from build123d import *

# Parameters (mm, degrees)
F1_DEPTH = 8
F2_R     = 1.5
F3_DEPTH = 3.8920101006
F4_R     = 0.5


with BuildPart() as f1:
    # F0 (on Front) → F1 (new body)
    with BuildSketch(Plane.XZ):
        with BuildLine():
            Line((3, 14.471053486), (0, 14.471053486))
            Line((0, 14.471053486), (0, -5.528946514))
            Line((0, -5.528946514), (3, -5.528946514))
            Line((3, -5.528946514), (3, -3.3778412531))
            ThreePointArc((3, -3.3778412531), (3.7830427709, -0.6913432113), (5.8869086913, 1.1536976821))
            Line((5.8869086913, 1.1536976821), (10.3150881731, 3.2185916862))
            Line((10.3150881731, 3.2185916862), (10.3150881731, -0.0229635164))
            Line((10.3150881731, -0.0229635164), (16.2366852164, -0.0229635164))
            Line((16.2366852164, -0.0229635164), (16.2366852164, 11.9770364836))
            Line((16.2366852164, 11.9770364836), (10.3150881731, 11.9770364836))
            Line((10.3150881731, 11.9770364836), (10.3150881731, 8.735481281))
            Line((10.3150881731, 8.735481281), (4.7242360053, 6.1284240995))
            ThreePointArc((4.7242360053, 6.1284240995), (3.5608002487, 6.2046797078), (3, 7.2268835811))
            Line((3, 7.2268835811), (3, 14.471053486))
        make_face()
    extrude(amount=F1_DEPTH)

    # F2 (on Right) → F3 (cut, through all)
    with BuildSketch(Plane.YZ):
        with Locations((-4, -2.028946514)):
            Circle(F2_R)
        with Locations((-4, 10.971053486)):
            Circle(F2_R)
    extrude(amount=F3_DEPTH, mode=Mode.SUBTRACT)

    # F4
    f4_edges = [f1.edges().sort_by_distance(p)[0] for p in [
        (7.519662, 0, 7.431953),
        (8.100998, 0, 2.186145),
        (7.519662, -8, 7.431953),
        (8.100998, -8, 2.186145),
    ]]
    fillet(f4_edges, radius=F4_R)


solid = f1.part
Model file for the job. Use its own axes, mm. A direction names the side the tool comes from. Give positions to 0.01 mm unless a question says otherwise; leave off trailing zeros. Write each loop counter-clockwise with the first axis right and the second up, starting at its lowest first coordinate (ties: lowest second). Pieces come first, ordered by that corner, then holes. Notation, with made-up numbers: (28, 41.25) - (55, 41.25) arc R22 ccw to (55, 73.25) - close; hole circle Ø3 at (58, -21.5). An arc over 180 degrees is marked (long way). Answer as CSV lines item,"result".
1. Band-saw the part on D-D (x = 2.75). Count the separate pieces of the cut face and the enclosed holes in it, and give its area (3 significant figures).
Responses:
separate pieces,"1"
enclosed holes,"2"
area,"144 mm2"
2. Band-saw the part on B-B (z = -3.75). Write the cut outline in (x, y).
Responses:
outline,"(0, -8) - (2.5, -8) arc R0.5 ccw to (3, -7.5) - (3, -0.5) arc R0.5 ccw to (2.5, 0) - (0, 0) - close"
3. Band-saw the part on A-A (y = -4). Write the cut outline in (x, z), and give its area (3 significant figures).
Responses:
outline,"(0, -5.53) - (3, -5.53) - (3, -3.53) - (0, -3.53) - close; (0, -0.53) - (3.89, -0.53) arc R5 cw to (5.89, 1.15) - (10.32, 3.22) - (10.32, -0.02) - (16.24, -0.02) - (16.24, 11.98) - (10.32, 11.98) - (10.32, 8.74) - (4.72, 6.13) arc R1.21 cw to (3, 7.23) - (3, 9.47) - (0, 9.47) - close; (0, 12.47) - (3, 12.47) - (3, 14.47) - (0, 14.47) - close"
area,"155 mm2"
4. Drill centre lines: L1, parallel to Z at x = 2.1, y = -4; L2, parallel to X at y = -6.5, z = 10.5; L3, parallel to Z at x = 15.75, y = -2.25. Where is each one in solid material? Low to high. Write a range as [from, to].
Responses:
L1,"z = [-5.53, -3.53], [-0.53, 9.47], [12.47, 14.47]"
L2,"x = [0, 3], [10.32, 16.24]"
L3,"z = [-0.02, 11.98]"
5. Band-saw the part on C-C (y = -5.75). Write the cut outline in (x, z), and give its area (3 significant figures).
Responses:
outline,"(0, -5.53) - (3, -5.53) - (3, -3.38) arc R5 cw to (5.89, 1.15) - (10.32, 3.22) - (10.32, -0.02) - (16.24, -0.02) - (16.24, 11.98) - (10.32, 11.98) - (10.32, 8.74) - (4.72, 6.13) arc R1.21 cw to (3, 7.23) - (3, 14.47) - (0, 14.47) - close"
area,"174 mm2"
6. 3-axis set-ups, long thin cutter, end or side, ignore diameter. For faces 4 (the face through (13, -4, 11.977)), 5 (the face through (13, -4, -0.023)), 6 (the face through (3, -6, 11)): which of +Z, -Z, +X, -X, +Y, -Y reach the whole face in a straight line?
Responses:
face 4,"+Z, +X, +Y, -Y"
face 5,"-Z, +X, +Y, -Y"
face 6,"+Z, +Y, -Y"
7. Pin check, flat tips, straight feed: pin 1 (3.5 mm diameter, centred on y = -4, z = 10.97, fed in from -X); pin 2 (4 mm diameter, centred on x = 13, y = -6, fed in from -Z); pin 3 (2.5 mm diameter, centred on y = -4.5, z = -4.5, fed in from +X). Stop position of each tip, or through.
Responses:
pin 1,"stops at x = 0"
pin 2,"stops at z = -0.02"
pin 3,"stops at x = 3"
8. Two-plate mould, pull along X, no slides. Class faces 1 (the face through (7.56, -3.95, 7.45)), 2 (the face through (3, -4, -4)), 3 (the face through (8, 0, 5)): +X half, -X half, draft (parallel to the pull), parting line (faces both ways), or undercut.
Responses:
face 1,"undercut"
face 2,"+X half"
face 3,"draft"
